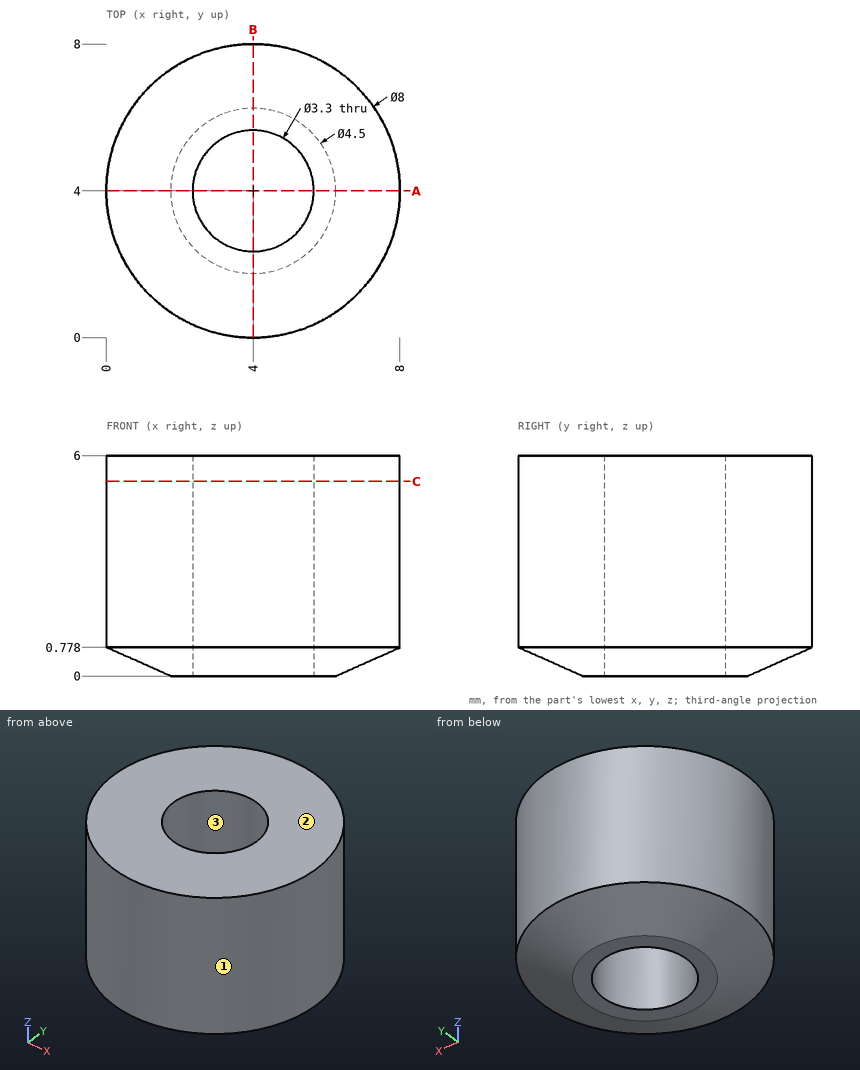
For this review, use the dimensioned drawing (mm, ordinates from the lowest corner) and the shaded views. Coordinates: 2 decimals unless noted, no trailing zeros. Loops run counter-clockwise (first coordinate to the right, second up) from the corner with the lowest first, then second, coordinate; pieces in that order, holes last. Notation, with made-up numbers: (14, 79.25) - (73, 79.25) arc R6 cw to (73, 83.25) - close; hole circle Ø2 at (50.5, -30). An arc over 180 degrees is marked (long way). Use one line per item in the form item = value. Start each with the question number.
1) Take a section at C-C (z = 5.3). State the section outline as (x, y) points, plus the area to 3 significant figures.
2) Draft analysis for pull direction X (two halves, no side actions). For the marked faces 1, 2 and 3, state which applies: released by +X, released by -X, zero draft, split by the parting line, or undercut.
3) Take a section at A-A (y = 4). State the section outline as (x, z) points.
4) To check wall thickness, follow probe 1 along Y at (x, z) = (4, 3.55); probe 2 along Y at (x, z) = (3, 5.3); probe 3 along X at (y, z) = (2.75, 4.8). State the ranges of each line that lie inside material, in increasing order. Write a range as from..to.
5) For pin 1 (1 mm diameter, centred on y = 5.5, z = 4.5, fed in from +X); pin 2 (2 mm diameter, centred on x = 1.5, z = 4, fed in from +Y); pin 3 (3 mm diameter, centred on x = 4, y = 4, fed in from +Z), all flat-tipped, find the tip position at first contact; note any pin that passes through.
From the geometry:
q1.outline = circle Ø8 at (4, 4); hole circle Ø3.3 at (4, 4)
q1.area = 41.7 mm2
q2.face_1 = split by the parting line
q2.face_2 = zero draft
q2.face_3 = undercut
q3.outline = (0, 0.78) - (1.75, 0) - (2.35, 0) - (2.35, 6) - (0, 6) - close; (5.65, 0) - (6.25, 0) - (8, 0.78) - (8, 6) - (5.65, 6) - close
q4.probe_1 = 0..2.35, 5.65..8
q4.probe_2 = 0.13..2.69, 5.31..7.87
q4.probe_3 = 0.2..2.92, 5.08..7.8
q5.pin_1 = 7.87
q5.pin_2 = 7.71
q5.pin_3 = through
